```python
from build123d import *

# Parameters (mm, degrees)
SKETCH_1_W          = 80
SKETCH_1_H          = 40
EXTRUDE_1_DEPTH     = 50
CUT_EXTRUDE_1_DEPTH = 76.498344353
SKETCH_3_R          = 4.5
CUT_EXTRUDE_2_DEPTH = 62.846584384


with BuildPart() as part:
    # 草图1 → 凸台-拉伸1 (new body)
    with BuildSketch(Plane.XY.offset(-25)):
        with Locations((0, 20)):
            Rectangle(SKETCH_1_W, SKETCH_1_H)
    extrude(amount=EXTRUDE_1_DEPTH)

    # 草图2 → 切除-拉伸1 (cut, through all)
    with BuildSketch(Plane.XY.offset(-25)):
        Polygon((-6, 40), (6, 40), (6, 30), (12, 30), (12, 22), (-12, 22), (-12, 30), (-6, 30), align=None)
    extrude(amount=CUT_EXTRUDE_1_DEPTH, mode=Mode.SUBTRACT)

    # 草图3 → 切除-拉伸2 (cut, through all)
    with BuildSketch(Plane(origin=(0, 40, 0), x_dir=(1, 0, 0), z_dir=(0, 1, 0))):
        with Locations(Location((-30, 0, 0), (0, 0, 270))):
            Circle(SKETCH_3_R)
        with Locations(Location((30, 0, 0), (0, 0, 270))):
            Circle(SKETCH_3_R)
    extrude(amount=-CUT_EXTRUDE_2_DEPTH, mode=Mode.SUBTRACT)


solid = part.part
```
Work out the finished part from the listing and answer in its coordinate system (mm). A direction names the side the tool comes from. Give positions to 0.01 mm unless a question says otherwise; leave off trailing zeros. Loops run counter-clockwise (first coordinate to the right, second up) from the corner with the lowest first, then second, coordinate; pieces in that order, holes last. Notation, with made-up numbers: (56.25, 2) -> (72.25, 2) arc R38 ccw to (72.25, 41) -> close; hole circle Ø4 at (26.25, -39). An arc over 180 degrees is marked (long way). Put each result on its own line as item: value. Start each with the question number.
Item 1: Find the intervals of material crossed by L1, parallel to X at y = 16.5, z = 0; L2, parallel to X at y = 29.5, z = 0; L3, parallel to X at y = 32.5, z = 0, in increasing order. Write a range as [from, to].
Item 2: The part is cut by section D-D (z = -6). Give the vertices of the cut face in (x, y), then the cut area to 3 significant figures.
Item 3: The part is cut by section A-A (y = 23.5). Give the vertices of the cut face in (x, z), then the cut area to 3 significant figures.
Item 4: The mould has two halves that part along X. Classify faces 4 (the face through (25.61, 20.28, -0.98)), 5 (the face through (40, 20, 0)), 6 (the face through (-23, 40, 0)): released by +X, released by -X, zero draft, split by the parting line, or undercut.
Item 5: The part is cut by section B-B (z = 0). Give the vertices of the cut face in (x, y).
Item 6: Which of the six approach directions +Z, -Z, +X, -X, +Y, -Y give full straight-line access (tool end or side, diameter ignored) to faces 1 (the face through (12, 26, 0)), 2 (the face through (23, 40, 0)), 3 (the face through (6, 35, 0))?
Item 7: Each of these flat-tipped pins is pushed along its axis until it touches: P1, Ø12, axis at x = -5, z = -10, coming from the +Y side; P2, Ø4, axis at x = 9.5, y = 27, coming from the -Z side. Where does it stop, or does it pass through?
Item 8: The part is cut by section C-C (x = 30). Give the vertices of the cut face in (y, z).
Answers below:
1. L1: [-40, -34.5], [-25.5, 25.5], [34.5, 40]
1. L2: [-40, -34.5], [-25.5, -12], [12, 25.5], [34.5, 40]
1. L3: [-40, -34.5], [-25.5, -6], [6, 25.5], [34.5, 40]
2. outline: (-40, 0) -> (40, 0) -> (40, 40) -> (6, 40) -> (6, 30) -> (12, 30) -> (12, 22) -> (-12, 22) -> (-12, 30) -> (-6, 30) -> (-6, 40) -> (-40, 40) -> close
2. area: 2,890 mm2
3. outline: (-40, -25) -> (-12, -25) -> (-12, 25) -> (-40, 25) -> close; (12, -25) -> (40, -25) -> (40, 25) -> (12, 25) -> close; hole circle Ø9 at (-30, 0); hole circle Ø9 at (30, 0)
3. area: 2,670 mm2
4. face 4: undercut
4. face 5: released by +X
4. face 6: zero draft
5. outline: (-40, 0) -> (-34.5, 0) -> (-34.5, 40) -> (-40, 40) -> close; (-25.5, 0) -> (25.5, 0) -> (25.5, 40) -> (6, 40) -> (6, 30) -> (12, 30) -> (12, 22) -> (-12, 22) -> (-12, 30) -> (-6, 30) -> (-6, 40) -> (-25.5, 40) -> close; (34.5, 0) -> (40, 0) -> (40, 40) -> (34.5, 40) -> close
6. face 1: +Z, -Z
6. face 2: +Z, -Z, +X, -X, +Y
6. face 3: +Z, -Z, +Y
7. P1: y = 40
7. P2: through
8. outline: (0, -25) -> (40, -25) -> (40, -4.5) -> (0, -4.5) -> close; (0, 4.5) -> (40, 4.5) -> (40, 25) -> (0, 25) -> close
